```python
from build123d import *
from build123d.topology import SkipClean

# Parameters (mm, degrees)
CROQUIS1_R                                     = 73.5
SALIENTE_EXTRUIR1_DEPTH                        = 5
CROQUIS7_R                                     = 73.5
CROQUIS7_R_2                                   = 61
SALIENTE_EXTRUIR2_DEPTH                        = 5
CROQUIS8_R                                     = 2.75
CORTAR_EXTRUIR5_DEPTH                          = 105.424613957
CORTAR_EXTRUIR6_DEPTH                          = 4
BOSS_EXTRUDE1_DEPTH                            = 2.5
CSK_SLOT_FOR_M3_FLAT_HEAD_MACHINE_SCREW1_DEPTH = 12.5
CIRPATTERN1_COUNT                              = 3
FILLET3_R                                      = 5


with BuildPart() as part:
    # Croquis1 → Saliente-Extruir1 (new body)
    with BuildSketch(Plane(origin=(0, 0, 0), x_dir=(1, 0, 0), z_dir=(0, 1, 0))):
        with Locations(Location((0, 0, 0), (0, 0, 270))):
            Circle(CROQUIS1_R)
    extrude(amount=SALIENTE_EXTRUIR1_DEPTH)

    # Croquis7 → Saliente-Extruir2 (add)
    with BuildSketch(Plane(origin=(0, 5, 0), x_dir=(1, 0, 0), z_dir=(0, 1, 0))):
        with Locations(Location((0, 0, 0), (0, 0, 270))):
            Circle(CROQUIS7_R)
        with Locations(Location((0, 0, 0), (0, 0, 270))):
            Circle(CROQUIS7_R_2, mode=Mode.SUBTRACT)
    extrude(amount=SALIENTE_EXTRUIR2_DEPTH)

    # Croquis8 → Cortar-Extruir5 (cut, through all)
    with BuildSketch(Plane(origin=(0, 10, 0), x_dir=(1, 0, 0), z_dir=(0, 1, 0))):
        with Locations(Location((-17.987923635, -67.131844927, 0), (0, 0, 270))):
            Circle(CROQUIS8_R)
        with Locations(Location((-67.131844927, 17.987923635, 0), (0, 0, 270))):
            Circle(CROQUIS8_R)
        with Locations(Location((17.987923635, 67.131844927, 0), (0, 0, 270))):
            Circle(CROQUIS8_R)
        with Locations(Location((67.131844927, -17.987923635, 0), (0, 0, 270))):
            Circle(CROQUIS8_R)
    extrude(amount=-CORTAR_EXTRUIR5_DEPTH, mode=Mode.SUBTRACT)

    # Croquis9 → Cortar-Extruir6 (cut)
    with BuildSketch(Plane(origin=(0, 0, 0), x_dir=(-1, 0, 0), z_dir=(0, -1, 0))):
        Polygon((20.297324711, -63.131844927), (15.678522558, -63.131844927), (13.369121481, -67.131844927), (15.678522558, -71.131844927), (20.297324711, -71.131844927), (22.606725788, -67.131844927), align=None)
        Polygon((-63.131844927, -20.297324711), (-63.131844927, -15.678522558), (-67.131844927, -13.369121481), (-71.131844927, -15.678522558), (-71.131844927, -20.297324711), (-67.131844927, -22.606725788), align=None)
        Polygon((-20.297324711, 63.131844927), (-15.678522558, 63.131844927), (-13.369121481, 67.131844927), (-15.678522558, 71.131844927), (-20.297324711, 71.131844927), (-22.606725788, 67.131844927), align=None)
        Polygon((63.131844927, 20.297324711), (63.131844927, 15.678522558), (67.131844927, 13.369121481), (71.131844927, 15.678522558), (71.131844927, 20.297324711), (67.131844927, 22.606725788), align=None)
    extrude(amount=-CORTAR_EXTRUIR6_DEPTH, mode=Mode.SUBTRACT)

    # Sketch3 → Boss-Extrude1 (add)
    with SkipClean():  # the faces are left unmerged after this step: merging them gives an invalid solid
        with BuildSketch(Plane(origin=(0, 10, 0), x_dir=(1, 0, 0), z_dir=(0, 1, 0))):
            with BuildLine():
                Line((11.696105723, 59.868197826), (11.869621272, 72.535247231))
                ThreePointArc((11.869621272, 72.535247231), (1.004194341, 73.493139773), (-9.883348207, 72.832475093))
                Line((-9.883348207, 72.832475093), (-10.056865919, 60.165267787))
                ThreePointArc((-10.056865919, 60.165267787), (0.832970242, 60.994312526), (11.696105723, 59.868197826))
            make_face()
            with BuildLine():
                Line((-57.695433057, -19.804974232), (-68.752177408, -25.98823006))
                ThreePointArc((-68.752177408, -25.98823006), (-64.149023218, -35.876912077), (-58.133099548, -44.975468168))
                Line((-58.133099548, -44.975468168), (-47.076217369, -38.792135262))
                ThreePointArc((-47.076217369, -38.792135262), (-53.239109255, -29.775782873), (-57.695433057, -19.804974232))
            make_face()
            with BuildLine():
                Line((45.999327335, -40.063223594), (56.882556136, -46.547017171))
                ThreePointArc((56.882556136, -46.547017171), (63.144828877, -37.616227696), (68.016447755, -27.857006925))
                Line((68.016447755, -27.857006925), (57.133083289, -21.373132525))
                ThreePointArc((57.133083289, -21.373132525), (52.406139013, -31.218529653), (45.999327335, -40.063223594))
            make_face()
        extrude(amount=BOSS_EXTRUDE1_DEPTH)

    # CSK SLOT for M3 Flat Head Machine Screw1: read off the stored shape, not the designer's step
    # CSK SLOT for M3 Flat Head Machine Sc 2 → CSK SLOT for M3 Flat Head Machine Screw1 (cut)
    with SkipClean():  # the faces are left unmerged after this step: merging them gives an invalid solid
        with BuildSketch(Plane(origin=(0, 0, 0), x_dir=(1, 0, 0), z_dir=(0, 1, 0))):
            with BuildLine():
                ThreePointArc((-60.230442327, -37.210480227), (-57.7715966, -37.869325954), (-57.112750874, -35.410480227))
                Line((-57.112750874, -35.410480227), (-60.167750874, -30.11906501))
                ThreePointArc((-60.167750874, -30.11906501), (-62.626596601, -29.460219283), (-63.285442327, -31.91906501))
                Line((-63.285442327, -31.91906501), (-60.230442327, -37.210480227))
            make_face()
        csk_slot_for_m3_flat_head_machine_screw1 = extrude(amount=CSK_SLOT_FOR_M3_FLAT_HEAD_MACHINE_SCREW1_DEPTH, mode=Mode.SUBTRACT)

    # CSK SLOT for M3 Flat Head Machine Sc 3: loft between two sections, ruled curve by curve
    with SkipClean():  # the faces are left unmerged after this step: merging them gives an invalid solid
        csk_slot_for_m3_flat_head_machine_sc_3_from = [
            Edge.make_three_point_arc((-57.112750874, 1.35, 35.410480227), (-56.932930113, 1.35, 36.776354508), (-57.7715966, 1.35, 37.869325954)),
            Edge.make_three_point_arc((-57.7715966, 1.35, 37.869325954), (-59.137470882, 1.35, 38.049146714), (-60.230442327, 1.35, 37.210480227)),
            Edge.make_three_point_arc((-63.285442327, 1.35, 31.91906501), (-63.465263088, 1.35, 30.553190729), (-62.6265966, 1.35, 29.460219283)),
            Edge.make_three_point_arc((-62.6265966, 1.35, 29.460219283), (-61.260722319, 1.35, 29.280398523), (-60.167750874, 1.35, 30.11906501)),
            Edge.make_line((-60.230442327, 1.35, 37.210480227), (-63.285442327, 1.35, 31.91906501)),
            Edge.make_line((-57.112750874, 1.35, 35.410480227), (-60.167750874, 1.35, 30.11906501)),
        ]
        csk_slot_for_m3_flat_head_machine_sc_3_to = [
            Edge.make_three_point_arc((-55.943616578, 0, 34.735480227), (-55.628930248, 0, 37.125760219), (-57.0965966, 0, 39.038460249)),
            Edge.make_three_point_arc((-57.0965966, 0, 39.038460249), (-59.486876592, 0, 39.35314658), (-61.399576622, 0, 37.885480227)),
            Edge.make_three_point_arc((-64.454576622, 0, 32.59406501), (-64.769262953, 0, 30.203785018), (-63.3015966, 0, 28.291084988)),
            Edge.make_three_point_arc((-63.3015966, 0, 28.291084988), (-60.911316608, 0, 27.976398657), (-58.998616578, 0, 29.44406501)),
            Edge.make_line((-61.399576622, 0, 37.885480227), (-64.454576622, 0, 32.59406501)),
            Edge.make_line((-55.943616578, 0, 34.735480227), (-58.998616578, 0, 29.44406501)),
        ]
        csk_slot_for_m3_flat_head_machine_sc_3 = Solid(Shell([*[Face.make_surface_from_curves(csk_slot_for_m3_flat_head_machine_sc_3_from[k], csk_slot_for_m3_flat_head_machine_sc_3_to[k]) for k in range(6)], Face(Wire(csk_slot_for_m3_flat_head_machine_sc_3_from)), Face(Wire(csk_slot_for_m3_flat_head_machine_sc_3_to))]))
        add(csk_slot_for_m3_flat_head_machine_sc_3, mode=Mode.SUBTRACT)

    # CirPattern1: CSK SLOT for M3 Flat Head Machine Screw1, CSK SLOT for M3 Flat Head Machine Sc 3 ×3 about axis
    with SkipClean():  # the faces are left unmerged after this step: merging them gives an invalid solid
        cirpattern1_axis = Axis((0, 0, 0), (0, 1, 0))
        add([csk_slot_for_m3_flat_head_machine_screw1.rotate(cirpattern1_axis, i * 360 / CIRPATTERN1_COUNT) for i in range(1, CIRPATTERN1_COUNT)], mode=Mode.SUBTRACT)
        add([csk_slot_for_m3_flat_head_machine_sc_3.rotate(cirpattern1_axis, i * 360 / CIRPATTERN1_COUNT) for i in range(1, CIRPATTERN1_COUNT)], mode=Mode.SUBTRACT)

    # Fillet3
    fillet3_edges = [part.edges().sort_by_distance(p)[0] for p in [
        (0, 5, -61),
    ]]
    fillet(fillet3_edges, radius=FILLET3_R - 0.0001)  # a hair under: the kernel refuses the full size


solid = part.part
```
Could you check a few things on this model? Use its own coordinates, in mm. A direction names the side the tool comes from. Round coordinates to 2 decimals unless told otherwise and drop trailing zeros. One line per question, with ' | ' between items. Start each with the question number.
(1) For P1, Ø4.5, axis at x = -18, y = 2.5, coming from the +Z side; P2, Ø1.5, axis at x = 33.5, y = 2.5, coming from the -Z side; P3, Ø2, axis at x = 22, z = -40.5, coming from the +Y side, each with a flat end and sliding along its axis, tell me the tip position at first contact or that it passes through.
(2) Please list where these lines run through material, in increasing order: line 1 along Z through (x, y) = (18, 5.5); line 2 along X through (y, z) = (9.75, -16.5); line 3 along Z through (x, y) = (0, 10.05).
(3) Thinking about a two-plate mould opening in X: for faces 1 (the face through (63.132, 2, 18)), 2 (the face through (-53, 10, -31)), which applies, +X half, -X half, draft (parallel to the pull), parting line (faces both ways), or undercut?
(4) For faces 3 (the face through (1, 0, -1)), 4 (the face through (-64, 4, -17)), 5 (the face through (51.365, 11.232, 43.26)), 6 (the face through (1, 7, -67.166)), which set-ups out of +Z, -Z, +X, -X, +Y, -Y let a thin tool reach every point of the face, with its end or its side?
(5) Suppose I cut it at B-B on y = 7.5. Count the separate pieces of the cut face and the enclosed holes in it, then the cut area to 3 significant figures.
Geometry results:
1) P1: z = 71.79 | P2: z = -65.8 | P3: y = 5
2) line 1: -71.26 to -69.88, -64.38 to -55.33, 55.33 to 71.26 | line 2: -71.62 to -69.44, -64.82 to -58.72, 58.72 to 71.62 | line 3: -73.5 to -70.77, -67.17 to -61
3) face 1: undercut | face 2: draft
4) face 3: +Z, -Z, +X, -X, -Y | face 4: -Y | face 5: +Z, +Y | face 6: +Y, -Y
5) separate pieces: 1 | enclosed holes: 8 | area: 5,350 mm²
